Read the model definition and answer for the solid it produces. Units are mm, in the model's axes. A direction names the side the tool comes from. Coordinates: 2 decimals unless noted, no trailing zeros. Write each loop counter-clockwise with the first axis right and the second up, starting at its lowest first coordinate (ties: lowest second). Pieces come first, ordered by that corner, then holes. Notation, with made-up numbers: (-18.75, 75.5) -> (9.25, 75.5) arc R19 ccw to (9.25, 109.5) -> close; hole circle Ø2 at (-0.5, -25). An arc over 180 degrees is marked (long way). Use CSV: the item, a comma, the result in double quotes. Start each with the question number.
from build123d import *

# Parameters (mm, degrees)
SKETCH1_R           = 15.748
EXTRUDE1_DEPTH      = 67.8688
CUT_EXTRUDE1_DEPTH  = 18.8976
SKETCH11_W          = 18.3134
SKETCH11_H          = 10.3251
S2D0011_W           = 4.5466
S2D0011_H           = 6.35
CUT_EXTRUDE10_DEPTH = 11.3538
EXTRUDE2_DEPTH      = 4.7752
CIRPATTERN2_COUNT   = 6
SKETCH18_W          = 11.3538
SKETCH18_H          = 0.127


with BuildPart() as part:
    # Sketch1 → Extrude1 (new body)
    with BuildSketch(Plane.XY):
        Circle(SKETCH1_R)
    extrude(amount=EXTRUDE1_DEPTH)

    # Sketch2 → Cut-Extrude1 (cut, symmetric)
    with BuildSketch(Plane(origin=(0, 0, 0), x_dir=(0, 0, 1), z_dir=(1, 0, 0))):
        with BuildLine():
            Line((58.7248, 15.748), (58.7248, 15.1638))
            ThreePointArc((58.7248, 15.1638), (58.992621559, 14.517221559), (59.6392, 14.2494))
            Line((59.6392, 14.2494), (67.8688, 14.2494))
            Line((67.8688, 14.2494), (67.8688, 15.748))
            Line((67.8688, 15.748), (58.7248, 15.748))
        make_face()
    cut_extrude1 = extrude(amount=CUT_EXTRUDE1_DEPTH, both=True, mode=Mode.SUBTRACT)

    # Sketch10 → Cut-Revolve1 (revolve, cut)
    with BuildSketch(Plane(origin=(0, 0, 0), x_dir=(0, 0, 1), z_dir=(1, 0, 0)), mode=Mode.PRIVATE) as cut_revolve1_sk:
        Polygon((0, 14.8717), (7.7978, 14.8717), (8.6741, 15.748), (0, 15.748), align=None)
    revolve(cut_revolve1_sk.sketch.rotate(Axis((0, 0, -0.433705), (0, 0, 1)), 90), axis=Axis((0, 0, -0.433705), (0, 0, 1)), mode=Mode.SUBTRACT)  # turned: the seam where the file's is

    # Sketch11 → Revolve1 (revolve)
    with BuildSketch(Plane(origin=(0, 0, 0), x_dir=(0, 0, -1), z_dir=(1, 0, 0)), mode=Mode.PRIVATE) as revolve1_sk:
        with Locations((-77.0255, 5.16255)):
            Rectangle(SKETCH11_W, SKETCH11_H)
    revolve(revolve1_sk.sketch.rotate(Axis((0, 0, 71.06412), (0, 0, -1)), 90), axis=Axis((0, 0, 71.06412), (0, 0, -1)))  # turned: the seam where the file's is

    # S2D0011 → Cut-Revolve2 (revolve, cut)
    with BuildSketch(Plane(origin=(-4.5466, 0, 70.3072), x_dir=(-1, 0, 0), z_dir=(0, 1, 0)), mode=Mode.PRIVATE) as cut_revolve2_sk:
        with Locations((-2.2733, 12.7)):
            Rectangle(S2D0011_W, S2D0011_H)
    revolve(cut_revolve2_sk.sketch.rotate(Axis((0, 0, 48.067068782), (0, 0, 1)), 180), axis=Axis((0, 0, 48.067068782), (0, 0, 1)), mode=Mode.SUBTRACT)  # turned: the seam where the file's is

    # Sketch14 → Cut-Extrude10 (cut)
    with BuildSketch(Plane.YX.offset(-86.1822)):
        with BuildLine():
            Line((-3.98523086, 9.525), (3.98523086, 9.525))
            ThreePointArc((3.98523086, 9.525), (0, 10.3251), (-3.98523086, 9.525))
        make_face()
        with BuildLine():
            Line((-3.98523086, -9.525), (3.98523086, -9.525))
            ThreePointArc((3.98523086, -9.525), (0, -10.3251), (-3.98523086, -9.525))
        make_face()
    extrude(amount=CUT_EXTRUDE10_DEPTH, mode=Mode.SUBTRACT)

    # Sketch15 → Extrude2 (add)
    with BuildSketch(Plane.XY.offset(86.1822)):
        Polygon((-4.582717762, 7.9375), (4.582717762, 7.9375), (9.165435523, 0), (4.582717762, -7.9375), (-4.582717762, -7.9375), (-9.165435523, 0), align=None)
    extrude(amount=EXTRUDE2_DEPTH)

    # Sketch16 → Cut-Revolve3 (revolve, cut)
    with BuildSketch(Plane(origin=(0, 0, 0), x_dir=(1, 0, 0), z_dir=(0, 1, 0))):
        Polygon((6.35, -90.9574), (9.165435523, -89.331907543), (9.165435523, -90.9574), align=None)
    revolve(axis=Axis((0, 0, 75.163674623), (0, 0, -1)), mode=Mode.SUBTRACT)

    # CirPattern2: Cut-Extrude1 ×6 about axis
    cirpattern2_axis = Axis((0, 0, 0), (0, 0, 1))
    for i in range(1, CIRPATTERN2_COUNT):
        add(cut_extrude1.rotate(cirpattern2_axis, i * 360 / CIRPATTERN2_COUNT), mode=Mode.SUBTRACT)

    # Sketch18 → Cut-Revolve4 (revolve, cut)
    with BuildSketch(Plane(origin=(0, 0, 0), x_dir=(0, 0, -1), z_dir=(1, 0, 0)), mode=Mode.PRIVATE) as cut_revolve4_sk:
        with Locations((-80.5053, 10.2616)):
            Rectangle(SKETCH18_W, SKETCH18_H)
    revolve(cut_revolve4_sk.sketch.rotate(Axis((0, 0, 0), (0, 0, 1)), 270), axis=Axis((0, 0, 0), (0, 0, 1)), mode=Mode.SUBTRACT)  # turned: the seam where the file's is


solid = part.part
1) Each of these flat-tipped pins is pushed along its axis until it touches: pin 1 (4 mm diameter, centred on x = 2, z = 80.5, fed in from +Y); pin 2 (10 mm diameter, centred on x = -7.5, z = 80, fed in from +Y); pin 3 (4.5 mm diameter, centred on x = 13, y = 8.5, fed in from +Z); pin 4 (4.5 mm diameter, centred on x = 0, y = -1, fed in from -Z). Where does it stop, or does it pass through?
2) Which of the six approach directions +Z, -Z, +X, -X, +Y, -Y give full straight-line access (tool end or side, diameter ignored) to faces 1 (the face through (12.39, -7.04, 63.7)), 2 (the face through (6.4, 5.2, 86.182)), 3 (the face through (6.862, -13.194, 3.953)), 4 (the face through (-12.39, 7.04, 63.7))?
3) Find the intervals of material crossed by line 1 along Z through (x, y) = (-1.5, -2); line 2 along Y through (x, z) = (0, 82); line 3 along Z through (x, y) = (-2, -11.5), in increasing order.
4) The mould has two halves that part along Y. Classify faces 5 (the face through (-6.91, 3.91, 88.08)), 6 (the face through (0, 0, 79.832)), 7 (the face through (13.3, 7.7, 58.725)): pulls with the +Y half, pulls with the -Y half, needs draft (parallel to the pull), parting line crosses it, or undercut.
5) Section B-B, the plane z = 10 is taken. Give the vertices of the cut face in (x, y).
The answers:
1,pin 1,"stops at y = 10.2"
1,pin 2,"stops at y = 9.89"
1,pin 3,"stops at z = 67.87"
1,pin 4,"stops at z = 0"
2,face 1,"+Z, +X, -Y"
2,face 2,"+Z"
2,face 3,"-Z"
2,face 4,"+Z, -X, +Y"
3,line 1,"z = 0 to 79.83, 86.18 to 90.96"
3,line 2,"y = -10.2 to -4.55, 4.55 to 10.2"
3,line 3,"z = 0 to 67.87"
4,face 5,"pulls with the +Y half"
4,face 6,"undercut"
4,face 7,"needs draft"
5,outline,"circle Ø31.5 at (0, 0)"
